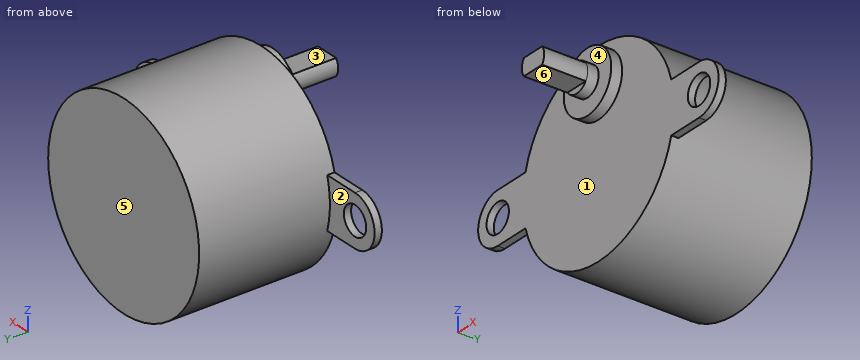
from build123d import *

# Parameters (mm, degrees)
SKETCH1_R           = 13.5
BOSS_EXTRUDE1_DEPTH = 19
SKETCH2_R           = 2
BOSS_EXTRUDE2_DEPTH = 1
SKETCH4_R           = 4.25
BOSS_EXTRUDE3_DEPTH = 1.5
SKETCH5_R           = 2
BOSS_EXTRUDE4_DEPTH = 1.5
BOSS_EXTRUDE5_DEPTH = 6


with BuildPart() as part:
    # Sketch1 → Boss-Extrude1 (new body)
    with BuildSketch(Plane(origin=(0, 0, 0), x_dir=(1, 0, 0), z_dir=(0, 1, 0))):
        Circle(SKETCH1_R)
    extrude(amount=BOSS_EXTRUDE1_DEPTH)

    # Sketch2 → Boss-Extrude2 (add)
    with BuildSketch(Plane.XZ):
        with BuildLine():
            Line((18, 3.5), (13.038405, 3.5))
            ThreePointArc((13.038405, 3.5), (13.5, 0), (13.038405, -3.5))
            Line((13.038405, -3.5), (18, -3.5))
            ThreePointArc((18, -3.5), (21.5, 0), (18, 3.5))
        make_face()
        with Locations((18, 0)):
            Circle(SKETCH2_R, mode=Mode.SUBTRACT)
    boss_extrude2 = extrude(amount=-BOSS_EXTRUDE2_DEPTH)

    # Mirror1: Boss-Extrude2 across plane
    add(boss_extrude2.mirror(Plane(origin=(0, 0, 0), x_dir=(0, 0, 1), z_dir=(1, 0, 0))))

    # Sketch4 → Boss-Extrude3 (add)
    with BuildSketch(Plane.XZ):
        with Locations((0, 8.5)):
            Circle(SKETCH4_R)
    extrude(amount=BOSS_EXTRUDE3_DEPTH)

    # Sketch5 → Boss-Extrude4 (add)
    with BuildSketch(Plane.XZ.offset(1.5)):
        with Locations((0, 8.5)):
            Circle(SKETCH5_R)
    extrude(amount=BOSS_EXTRUDE4_DEPTH)

    # Sketch6 → Boss-Extrude5 (add)
    with BuildSketch(Plane.XZ.offset(3)):
        with BuildLine():
            Line((-1.636307, 9.65), (1.636307, 9.65))
            ThreePointArc((1.636307, 9.65), (2, 8.5), (1.636307, 7.35))
            Line((1.636307, 7.35), (-1.636307, 7.35))
            ThreePointArc((-1.636307, 7.35), (-2, 8.5), (-1.636307, 9.65))
        make_face()
    extrude(amount=BOSS_EXTRUDE5_DEPTH)


solid = part.part
For this review, take the finished solid that the model builds, in its own axes (mm). Face numbers are marked on the shaded views. A direction names the side the tool comes from. Round coordinates to 2 decimals unless told otherwise and drop trailing zeros. Order: outer loops, then holes, each group sorted by start corner. A loop starts at its lowest first (then second) coordinate and runs counter-clockwise, first axis right, second up. Notation, with made-up numbers: M -22.5,-9.5 L -15.5,-9.5 A30 ccw -15.5,24.5 Z; hole C 43,-20 d11. An arc over 180 degrees is marked long. Write each question's results on one line, items separated by ' | '. Start each with the question number.
1. Add section D-D (z = 8.5). State the section outline as (x, y) points, then the cut area to 3 significant figures.
2. Tool access review of the marked faces 4, 5 and 6: name each direction out of +Z, -Z, +X, -X, +Y, -Y from which nothing blocks a thin tool from reaching the whole face with its end or side.
3. To check wall thickness, follow L1, parallel to Z at x = -18, y = 0.3; L2, parallel to X at y = -7.25, z = 8.5; L3, parallel to Y at x = 11, z = -7. State the ranges of each line that lie inside material, in increasing order. Write a range as [from, to].
4. Add section B-B (x = 0). State the section outline as (y, z) points, then the cut area to 3 significant figures.
5. Clearance check with flat-ended pins moving along their axes: pin 1 Ø13.5 at (x, z) = (-0.5, -0.5) entering from -Y; pin 2 Ø10 at (x, y) = (14.5, 0) entering from +Z; pin 3 Ø1.5 at (x, y) = (-0.5, 14) entering from -Z; pin 4 Ø5 at (y, z) = (14, 4.5) entering from -X. State where each tip first meets the part, or that it passes through.
6. Draft analysis for pull direction Y (two halves, no side actions). For the marked faces 1, 2 and 3, state which applies: pulls with the +Y half, pulls with the -Y half, needs draft (parallel to the pull), parting line crosses it, or undercut.
7. Add section C-C (x = 18.5). State the section outline as (y, z) points, then the cut area to 3 significant figures.
8. Add section A-A (z = 0). State the section outline as (x, y) points, then the cut area to 3 significant figures.
Output values:
1) outline: M -10.49,0 L -4.25,0 L -4.25,-1.5 L -2,-1.5 L -2,-9 L 2,-9 L 2,-1.5 L 4.25,-1.5 L 4.25,0 L 10.49,0 L 10.49,19 L -10.49,19 Z | area: 441 mm^2
2) face 4: -Y | face 5: +Z, -Z, +X, -X, +Y | face 6: -Z, +X, -X, -Y
3) L1: [-3.5, -2], [2, 3.5] | L2: [-2, 2] | L3: [0, 19]
4) outline: M -9,7.35 L -3,7.35 L -3,6.5 L -1.5,6.5 L -1.5,4.25 L 0,4.25 L 0,-13.5 L 19,-13.5 L 19,13.5 L 0,13.5 L 0,12.75 L -1.5,12.75 L -1.5,10.5 L -3,10.5 L -3,9.65 L -9,9.65 Z | area: 546 mm^2
5) pin 1: y = -1.5 | pin 2: z = 9.59 | pin 3: z = -13.5 | pin 4: x = -13.35
6) face 1: pulls with the -Y half | face 2: pulls with the +Y half | face 3: needs draft
7) outline: M 0,-3.46 L 1,-3.46 L 1,-1.94 L 0,-1.94 Z; M 0,1.94 L 1,1.94 L 1,3.46 L 0,3.46 Z | area: 3.06 mm^2
8) outline: M -21.5,0 L -20,0 L -20,1 L -21.5,1 Z; M -16,0 L 16,0 L 16,1 L 13.5,1 L 13.5,19 L -13.5,19 L -13.5,1 L -16,1 Z; M 20,0 L 21.5,0 L 21.5,1 L 20,1 Z | area: 521 mm^2
